Geometry: final body of the model. Coordinates: model frame, mm. Face numbers are marked on the shaded views. A direction names the side the tool comes from. Give positions to 0.01 mm unless a question says otherwise; leave off trailing zeros. Loops run counter-clockwise (first coordinate to the right, second up) from the corner with the lowest first, then second, coordinate; pieces in that order, holes last.
1. Material intervals for line 1 along Z through (x, y) = (39.5, 16); line 2 along Y through (x, z) = (31, 34), sorted ascending.
2. Access query for the marked faces 1, 2 and 3. Directions: +Z, -Z, +X, -X, +Y, -Y. A direction counts if a zero-diameter tool reaches every point of the face in a straight line with its end or side. Return the directions, or none.
3. First-contact query: P1, Ø10, axis at x = 31, z = 31.5, coming from the -Y side; P2, Ø8, axis at x = 23.5, y = 11, coming from the +Z side; P3, Ø10, axis at y = 20.5, z = 30, coming from the -X side; P4, Ø8, axis at x = 42.5, z = 7, coming from the -Y side. Flat tips, straight axial feed; report the tip coordinate or a pass-through.
4. Section A-A, the plane x = 37. Output: boundary loops of the cut face in (y, z), then the cut area to 3 significant figures.
5. Section B-B, the plane y = 16. Output: boundary loops of the cut face in (x, z).
6. Section D-D, the plane y = 29. Output: boundary loops of the cut face in (x, z).
7. Section C-C, the plane x = 5.5. Output: boundary loops of the cut face in (y, z).
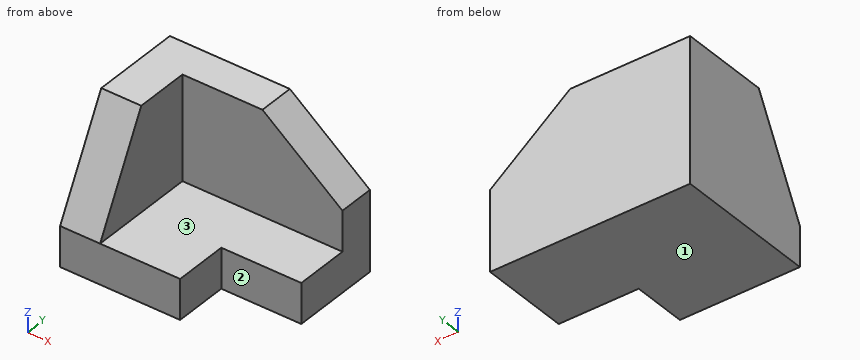
from build123d import *

# Parameters (mm, degrees)
F1_DEPTH = 36
F2_DEPTH = 27
F4_DEPTH = 10.001
F5_W     = 20
F5_H     = 13.5
F6_DEPTH = 10.001


with BuildPart() as f1:
    # F0 (on Front) → F1 (new body)
    with BuildSketch(Plane.XZ):
        Polygon((0, 36), (0, 0), (50, 0), (50, 10), (10, 10), (10, 36), align=None)
        Polygon((10, 10), (50, 10), (50, 20), (30, 36), (10, 36), align=None)
    extrude(amount=-F1_DEPTH)

    # F0 (on Front) → F2 (cut)
    with BuildSketch(Plane.XZ):
        Polygon((10, 10), (50, 10), (50, 20), (30, 36), (10, 36), align=None)
    extrude(amount=-F2_DEPTH, mode=Mode.SUBTRACT)

    # F3 (on face) → F4 (cut, through all)
    with BuildSketch(Plane.YZ.offset(10)):
        Polygon((0, 10), (13.5, 36), (0, 36), align=None)
    extrude(amount=-F4_DEPTH, mode=Mode.SUBTRACT)

    # F5 (on face) → F6 (cut, through all)
    with BuildSketch(Plane.XY.offset(10)):
        with Locations((40, 6.75)):
            Rectangle(F5_W, F5_H)
    extrude(amount=-F6_DEPTH, mode=Mode.SUBTRACT)


solid = f1.part
Answers below:
1. line 1: z = 0 to 10
1. line 2: y = 27 to 36
2. face 1: -Z, +X, -X, +Y, -Y
2. face 2: +Z, -Z, +X, -Y
2. face 3: +Z, +X, -Y
3. P1: stops at y = 27
3. P2: stops at z = 10
3. P3: stops at x = 0
3. P4: stops at y = 13.5
4. outline: (13.5, 0) - (36, 0) - (36, 30.4) - (27, 30.4) - (27, 10) - (13.5, 10) - close
4. area: 409 mm2
5. outline: (0, 0) - (50, 0) - (50, 10) - (10, 10) - (10, 36) - (0, 36) - close
6. outline: (0, 0) - (50, 0) - (50, 20) - (30, 36) - (0, 36) - close
7. outline: (0, 0) - (36, 0) - (36, 36) - (13.5, 36) - (0, 10) - close
